The model under review builds one solid part; all positions refer to its coordinate system, in mm. Round coordinates to 2 decimals unless told otherwise and drop trailing zeros. Order: outer loops, then holes, each group sorted by start corner. A loop starts at its lowest first (then second) coordinate and runs counter-clockwise, first axis right, second up. Notation, with made-up numbers: M -3,27 L 13,27 A6 cw 13,31 Z; hole C 35.5,-14.5 d6. An arc over 180 degrees is marked long. One line per item, written item: value. Start each with the question number.
from build123d import *

# Parameters (mm, degrees)
EXTRUDE1_DEPTH         = 0.127
SKETCH4_W              = 0.508
SKETCH4_H              = 0.3048
SKETCH4_W_2            = 0.762
SKETCH4_H_2            = 0.508
EB_02_TAB_1_DEPTH      = 0.127
SKETCH2_W              = 0.762
SKETCH2_H              = 0.5588
EB_02_TAB_2_DEPTH      = 0.127
LP_01_TAB_2_X_18_COUNT = 18
LP_01_TAB_2_X_18_PITCH = 5.08


with BuildPart() as part:
    # Sketch1 → Extrude1 (new, symmetric)
    with BuildSketch(Plane.XY):
        Polygon((16.891, 0), (131.6228, 0), (131.6228, -5.171473897), (16.891, -0.663649197), align=None)
    extrude(amount=EXTRUDE1_DEPTH, both=True)

    # Sketch4 → EB-02 Tab 1 (add, symmetric)
    with BuildSketch(Plane.XY):
        with Locations((17.145, 0.1524)):
            Rectangle(SKETCH4_W, SKETCH4_H)
        with Locations((29.6164, 0.0508)):
            Rectangle(SKETCH4_W_2, SKETCH4_H_2)
    extrude(amount=EB_02_TAB_1_DEPTH, both=True)

    # Sketch2 → EB-02 Tab 2 (add, symmetric)
    with BuildSketch(Plane.XY):
        with Locations((39.37, 0.0254)):
            Rectangle(SKETCH2_W, SKETCH2_H)
    eb_02_tab_2 = extrude(amount=EB_02_TAB_2_DEPTH, both=True)

    # LP-01 Tab 2 x 18: EB-02 Tab 2 ×18
    with Locations(*[(i * LP_01_TAB_2_X_18_PITCH, 0, 0) for i in range(1, LP_01_TAB_2_X_18_COUNT)]):
        add(eb_02_tab_2)


solid = part.part
Item 1: Consider section B-B, the plane x = 72.5. Give the boundary of the cut face in (y, z).
Item 2: Wall thickness on L1, parallel to Y at x = 50, z = -0.05; L2, parallel to Y at x = 32.5, z = 0: over which ranges is each line inside the solid? List them lowest first.
Item 3: Consider section A-A, the plane y = -3.2. Give the boundary of the cut face in (x, z), then the cut area to 3 significant figures.
Computed:
1. outline: M -2.85,-0.13 L 0,-0.13 L 0,0.13 L -2.85,0.13 Z
2. L1: y = -1.96 to 0
2. L2: y = -1.28 to 0
3. outline: M 81.45,-0.13 L 131.62,-0.13 L 131.62,0.13 L 81.45,0.13 Z
3. area: 12.7 mm^2
